```python
from build123d import *

# Parameters (mm, degrees)
SKETCH_1_W               = 50
SKETCH_1_H               = 50
EXTRUDE_1_DEPTH          = 16
SKETCH_3_R               = 1.6
CUT_EXTRUDE_1_DEPTH      = 39.807215824
SKETCH_6_W               = 25
SKETCH_6_H               = 12
CUT_EXTRUDE_3_DEPTH      = 12
SKETCH_7_R               = 2.55
CUT_EXTRUDE_4_DEPTH      = 15.1
PATTERN_CIRCULAR_2_COUNT = 4
SKETCH_8_W               = 50
SKETCH_8_H               = 50
CUT_EXTRUDE_5_DEPTH      = 8


with BuildPart() as part:
    # 草图1 → 凸台-拉伸1 (new body)
    with BuildSketch(Plane(origin=(0, 0, 0), x_dir=(1, 0, 0), z_dir=(0, 1, 0))):
        Rectangle(SKETCH_1_W, SKETCH_1_H)
    extrude(amount=EXTRUDE_1_DEPTH)

    # 草图2 → 切除-旋转1 (revolve, cut)
    with BuildSketch(Plane.XY):
        with BuildLine():
            Line((0, 18), (0, -2))
            ThreePointArc((0, -2), (10, 8), (0, 18))
        make_face()
    revolve(axis=Axis((0, 16, 0), (0, -1, 0)), mode=Mode.SUBTRACT)

    # 草图3 → 切除-拉伸1 (cut, through all)
    with BuildSketch(Plane(origin=(0, 16, 0), x_dir=(1, 0, 0), z_dir=(0, 1, 0))):
        with Locations(Location((-21, 21, 0), (0, 0, 270))):
            Circle(SKETCH_3_R)
        with Locations(Location((21, 21, 0), (0, 0, 270))):
            Circle(SKETCH_3_R)
        with Locations(Location((21, -21, 0), (0, 0, 270))):
            Circle(SKETCH_3_R)
        with Locations(Location((-21, -21, 0), (0, 0, 270))):
            Circle(SKETCH_3_R)
    extrude(amount=-CUT_EXTRUDE_1_DEPTH, mode=Mode.SUBTRACT)

    # 草图6 → 切除-拉伸3 (cut)
    with BuildSketch(Plane.XY.offset(25)):
        with Locations((0, 8)):
            Rectangle(SKETCH_6_W, SKETCH_6_H)
    cut_extrude_3 = extrude(amount=-CUT_EXTRUDE_3_DEPTH, mode=Mode.SUBTRACT)

    # 草图7 → 切除-拉伸4 (cut, symmetric)
    with BuildSketch(Plane(origin=(0, 0, 0), x_dir=(0, 0, -1), z_dir=(1, 0, 0))):
        with Locations(Location((-19.5, 8, 0), (0, 0, 180))):
            Circle(SKETCH_7_R)
    cut_extrude_4 = extrude(amount=CUT_EXTRUDE_4_DEPTH, both=True, mode=Mode.SUBTRACT)

    # 阵列(圆周)2: 切除-拉伸3, 切除-拉伸4 ×4 about axis
    pattern_circular_2_axis = Axis((0, 0, 0), (0, 1, 0))
    add([cut_extrude_3.rotate(pattern_circular_2_axis, i * 360 / PATTERN_CIRCULAR_2_COUNT) for i in range(1, PATTERN_CIRCULAR_2_COUNT)], mode=Mode.SUBTRACT)
    add([cut_extrude_4.rotate(pattern_circular_2_axis, i * 360 / PATTERN_CIRCULAR_2_COUNT) for i in range(1, PATTERN_CIRCULAR_2_COUNT)], mode=Mode.SUBTRACT)

    # 草图8 → 切除-拉伸5 (cut)
    with BuildSketch(Plane(origin=(0, 16, 0), x_dir=(1, 0, 0), z_dir=(0, 1, 0))):
        Rectangle(SKETCH_8_W, SKETCH_8_H)
    extrude(amount=-CUT_EXTRUDE_5_DEPTH, mode=Mode.SUBTRACT)


solid = part.part
```
The listing builds one solid part. Answer for the finished solid, in the listing's coordinates (mm). A direction names the side the tool comes from. Give positions to 0.01 mm unless a question says otherwise; leave off trailing zeros. Write each loop counter-clockwise with the first axis right and the second up, starting at its lowest first coordinate (ties: lowest second). Pieces come first, ordered by that corner, then holes. Notation, with made-up numbers: M 22.5,35.25 L 58.5,35.25 A13 ccw 58.5,44.25 Z; hole C 16.25,85.5 d11. An arc over 180 degrees is marked long. Write each question's results on one line, items separated by ' | '.
Q1. Section C-C, the plane x = -8 is taken. Write down the section's boundary in (y, z), then the cut area to 3 significant figures.
Output values:
outline: M 0,-25 L 2,-25 L 2,-13 L 8,-13 L 8,-6 A6 cw 8,6 L 8,13 L 2,13 L 2,25 L 0,25 Z | area: 199 mm2
Q2. Flat-ended cylindrical pins translate along their axes: P1, Ø3, axis at y = 4, z = 1.5, coming from the -X side; P2, Ø9.5, axis at x = -21, z = -3.5, coming from the +Y side; P3, Ø4, axis at x = 9, y = 7, coming from the +Z side. Find the tip coordinate at first contact, or state that the pin passes through.
Output values:
P1: x = -13 | P2: y = 2 | P3: z = 13
Q3. A tool of negligible diameter and unlimited length cuts with its end or side. For faces 4 (the flat face through (-12.5, 4, -19)), 5 (the flat face through (0, 5, 13)), 6 (the cylindrical face through (-13.82, 5.45, -19.56)), from which of +Z, -Z, +X, -X, +Y, -Y can it reach the whole face along a straight path? Write none if from no direction.
Output values:
face 4: -Z, +Y | face 5: +Z, +Y | face 6: +Y
Q4. For a pull along Z with two mould halves and no side action, classify faces 1 (the flat face through (0, 5, -13)), 2 (the cylindrical face through (-19.56, 5.45, 13.82)), 3 (the flat face through (0, 8, -11)) as released by +Z, released by -Z, zero draft, split by the parting line, or undercut.
Output values:
face 1: released by -Z | face 2: undercut | face 3: zero draft
Q5. Section A-A, the plane x = 21 is taken. Write down the section's boundary in (y, z).
Output values:
outline: M 0,-25 L 8,-25 L 8,-22.6 L 0,-22.6 Z; M 0,-19.4 L 8,-19.4 L 8,-15.1 L 5.94,-15.1 L 5.94,-12.5 L 2,-12.5 L 2,12.5 L 5.94,12.5 L 5.94,15.1 L 8,15.1 L 8,19.4 L 0,19.4 Z; M 0,22.6 L 8,22.6 L 8,25 L 0,25 Z
Q6. Section D-D, the plane z = -9 is taken. Write down the section's boundary in (x, y), then the cut area to 3 significant figures.
Output values:
outline: M -25,0 L 25,0 L 25,2 L 13,2 L 13,8 L 4.36,8 A4.36 cw -4.36,8 L -13,8 L -13,2 L -25,2 Z | area: 226 mm2
Q7. Section B-B, the plane z = 21 is taken. Write down the section's boundary in (x, y), then the cut area to 3 significant figures.
Output values:
outline: M -25,0 L -22.6,0 L -22.6,8 L -25,8 Z; M -19.4,0 L 19.4,0 L 19.4,8 L 15.1,8 L 15.1,5.94 L 12.5,5.94 L 12.5,2 L -12.5,2 L -12.5,5.94 L -15.1,5.94 L -15.1,8 L -19.4,8 Z; M 22.6,0 L 25,0 L 25,8 L 22.6,8 Z | area: 188 mm2
Q8. Consider L1, parallel to X at y = 3.75, z = -21; L2, parallel to X at y = 4.75, z = 18; L3, parallel to Z at x = 18.5, y = 6.25. Determine where each line is inside the solid, lowest interval first. Write a range as from..to.
Output values:
L1: -25..-22.6, -19.4..-12.5, 12.5..19.4, 22.6..25 | L2: -25..-12.5, 12.5..25 | L3: -25..-15.1, 15.1..25
